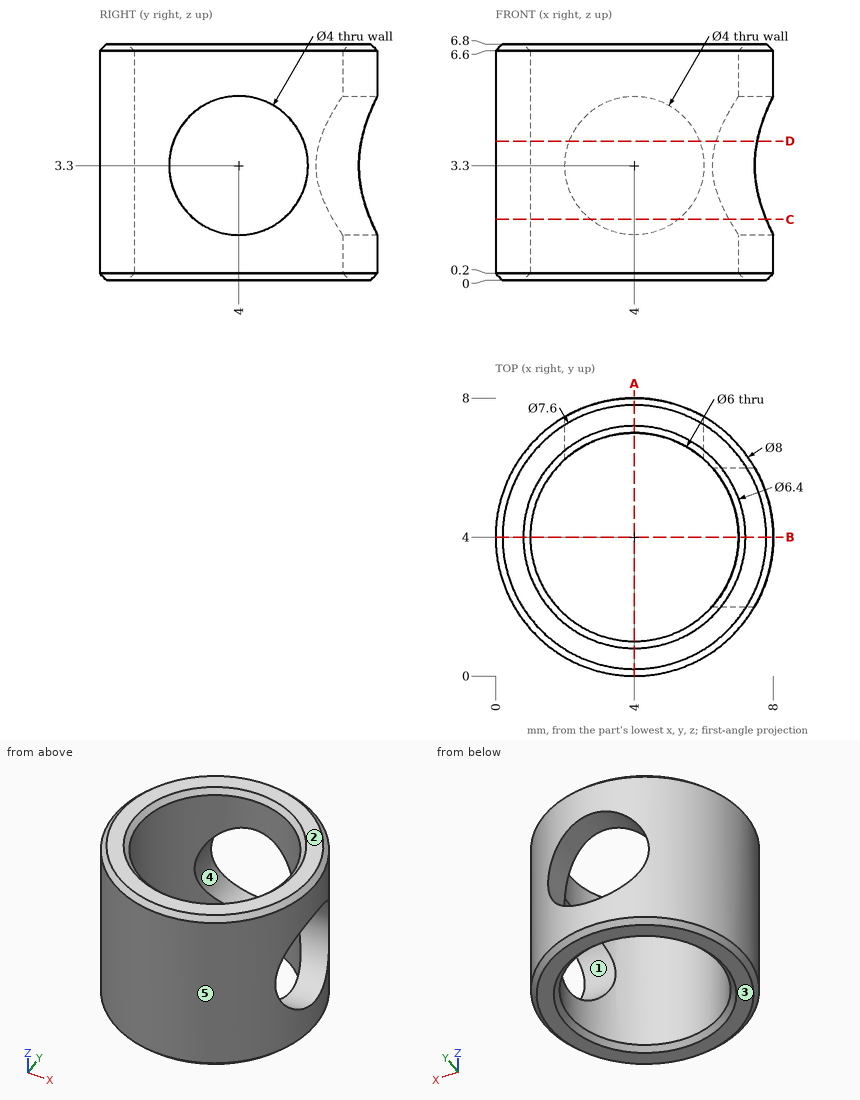
Job drawing, mm, ordinate dimensions from the low corner. One solid piece. A direction names the side the tool comes from. Round coordinates to 2 decimals unless told otherwise and drop trailing zeros. Order: outer loops, then holes, each group sorted by start corner. A loop starts at its lowest first (then second) coordinate and runs counter-clockwise, first axis right, second up. Notation, with made-up numbers: (-26.5, -31.5) -> (-7.5, -31.5) arc R28 ccw to (-7.5, -6.5) -> close; hole circle Ø2 at (10.25, 16.5). An arc over 180 degrees is marked (long way). Write item = value, one per line.
(1) Flat gauge pins, fed straight in: P1, Ø1, axis at x = 1, z = 5.5, coming from the -Y side; P2, Ø1, axis at y = 6, z = 3.5, coming from the -X side. Where does each tip first touch, or does it go through?
Answers follow:
P1 = 0.88
P2 = 0.29
(2) 3-axis set-ups, long thin cutter, end or side, ignore diameter. For the marked faces 4 and 5: which of +Z, -Z, +X, -X, +Y, -Y reach the whole face in a straight line?
Answers follow:
face_4 = +Y
face_5 = +Z, -Z
(3) Cut at C-C (z = 1.75). Write the cut outline in (x, y).
Answers follow:
outline = (2.74, 6.72) -> (2.74, 7.8) arc R4 ccw (long way) to (7.8, 2.74) -> (6.72, 2.74) arc R3 cw (long way) to start; (5.26, 6.72) arc R3 cw to (6.72, 5.26) -> (7.8, 5.26) arc R4 ccw to (5.26, 7.8) -> close
(4) Cut at A-A (x = 4). Write the cut outline in (y, z), plus the area to 3 significant figures.
Answers follow:
outline = (0, 0.2) -> (0.2, 0) -> (0.8, 0) -> (1, 0.2) -> (1, 6.6) -> (0.8, 6.8) -> (0.2, 6.8) -> (0, 6.6) -> close; (7, 0.2) -> (7.2, 0) -> (7.8, 0) -> (8, 0.2) -> (8, 1.3) -> (7, 1.3) -> close; (7, 5.3) -> (8, 5.3) -> (8, 6.6) -> (7.8, 6.8) -> (7.2, 6.8) -> (7, 6.6) -> close
area = 9.44 mm²
(5) Cut at D-D (z = 4). Write the cut outline in (x, y).
Answers follow:
outline = (2.13, 6.34) -> (2.13, 7.53) arc R4 ccw (long way) to (7.53, 2.13) -> (6.34, 2.13) arc R3 cw (long way) to start; (5.87, 6.34) arc R3 cw to (6.34, 5.87) -> (7.53, 5.87) arc R4 ccw to (5.87, 7.53) -> close
(6) Pull direction Z, two halves, no side cores. Call the marked faces 1, 2 and 3: +Z half, -Z half, draft (parallel to the pull), parting line (faces both ways), or undercut.
Answers follow:
face_1 = undercut
face_2 = +Z half
face_3 = -Z half
(7) Drill centre lines: L1, parallel to Z at x = 4.5, y = 7; L2, parallel to X at y = 7.2, z = 3.3; L3, parallel to X at y = 6.7, z = 3.3. Where is each one in solid material? Low to high.
Answers follow:
L1 = 0.16 to 1.36, 5.24 to 6.64
L2 = 1.6 to 2, 6 to 6.4
L3 = 1.05 to 2, 6 to 6.95
